Here's how the part is built. I have some questions about the finished solid (model axes, mm). Face numbers are marked on the shaded views. A direction names the side the tool comes from. Give positions to 0.01 mm unless a question says otherwise; leave off trailing zeros. Write each loop counter-clockwise with the first axis right and the second up, starting at its lowest first coordinate (ties: lowest second). Pieces come first, ordered by that corner, then holes. Notation, with made-up numbers: (67, 45.5) -> (122, 45.5) arc R19 cw to (122, 49.5) -> close; hole circle Ø4 at (-10, 45). An arc over 180 degrees is marked (long way). Return JSON: item names as keys, results as strings.
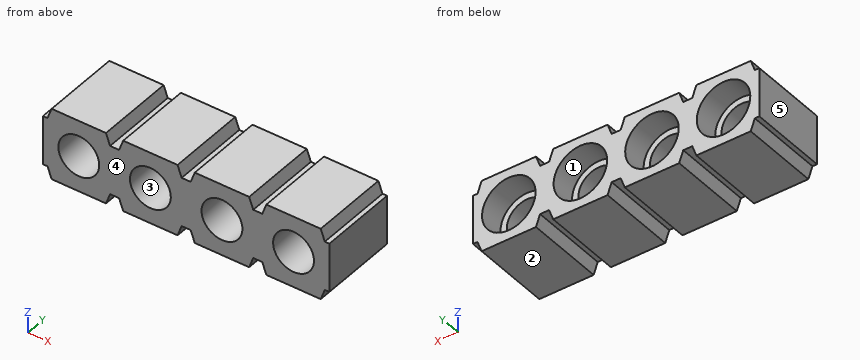
from build123d import *

# Parameters (mm, degrees)
EXTRUDE1_DEPTH    = 2.794
HOLE1_D           = 1.45034
HOLE1_CBORE_D     = 1.89992
HOLE1_CBORE_DEPTH = 0.89408
EXTRUDE2_DEPTH    = 2.794
LPATTERN1_COUNT   = 4
LPATTERN1_PITCH   = 2.54
LPATTERN2_COUNT   = 63
LPATTERN2_PITCH   = 2.54


with BuildPart() as part:
    # Sketch1 → Extrude1 (new body)
    with BuildSketch(Plane(origin=(0, 0, 0), x_dir=(1, 0, 0), z_dir=(0, 1, 0))):
        Polygon((9.854373708, 0.40005), (9.694353708, 0.40005), (9.548747416, 0), (0, 0), (-0.145606292, 0.40005), (-0.305626292, 0.40005), (-0.305626292, 2.13995), (-0.145606292, 2.13995), (0, 2.54), (9.548747416, 2.54), (9.694353708, 2.13995), (9.854373708, 2.13995), align=None)
    extrude(amount=-EXTRUDE1_DEPTH)

    # Hole1 (through all)
    with Locations(Plane(origin=(0.964373708, 0, -1.27), x_dir=(0, 0, 1), z_dir=(0, 1, 0))):
        with Locations((0, 0)):
            hole1 = CounterBoreHole(HOLE1_D / 2, HOLE1_CBORE_D / 2, HOLE1_CBORE_DEPTH)

    # Sketch4 → Extrude2 (cut)
    with BuildSketch(Plane(origin=(0, 0, 0), x_dir=(1, 0, 0), z_dir=(0, 1, 0))):
        Polygon((1.928772816, 0), (2.5399746, 0), (2.394368308, 0.40005), (2.074379108, 0.40005), align=None)
        Polygon((2.074379108, 2.13995), (2.394368308, 2.13995), (2.5399746, 2.54), (1.928772816, 2.54), align=None)
    extrude2 = extrude(amount=-EXTRUDE2_DEPTH, mode=Mode.SUBTRACT)

    # LPattern1: Hole1 ×4
    with Locations(*[(i * LPATTERN1_PITCH, 0, 0) for i in range(1, LPATTERN1_COUNT)]):
        add(hole1, mode=Mode.SUBTRACT)

    # LPattern2: Extrude2 ×63
    with Locations(*[(i * LPATTERN2_PITCH, 0, 0) for i in range(1, LPATTERN2_COUNT)]):
        add(extrude2, mode=Mode.SUBTRACT)


solid = part.part
1. For pin 1 Ø1.5 at (x, z) = (1, -1.5) entering from +Y; pin 2 Ø0.9 at (x, z) = (8.58, -1.27) entering from +Y, each with a flat end and sliding along its axis, tell me the tip position at first contact or that it passes through.
Taken from the geometry:
{"pin 1": "stops at y = 0", "pin 2": "passes through"}
2. If I drill on line 1 (X direction, y = -0.7, z = -1.27); line 2 (X direction, y = -2.05, z = -1.27); line 3 (X direction, y = -2.6, z = -2.3), over which ranges is the centre line in solid material (lowest first)? Write a range as [from, to].
Taken from the geometry:
{"line 1": "x = [-0.31, 0.01], [1.91, 2.55], [4.45, 5.09], [6.99, 7.63], [9.53, 9.85]", "line 2": "x = [-0.31, 0.24], [1.69, 2.78], [4.23, 5.32], [6.77, 7.86], [9.31, 9.85]", "line 3": "x = [-0.09, 2.02], [2.45, 4.56], [4.99, 7.1], [7.53, 9.64]"}
3. Which directions (+Z, -Z, +X, -X, +Y, -Y) give clear straight access to the entire face, cutting with the end or side of a thin tool? Please do the marked faces 1 and 2.
Taken from the geometry:
{"face 1": "+Y", "face 2": "-Z, +X, -X, +Y, -Y"}
4. Suppose I cut it at D-D, the plane x = 0.5. List the corners of the cut face in (y, z) for me, and give its area (3 significant figures).
Taken from the geometry:
{"outline": "(-2.79, -2.54) -> (0, -2.54) -> (0, -2.1) -> (-0.89, -2.1) -> (-0.89, -1.83) -> (-2.79, -1.83) -> close; (-2.79, -0.71) -> (-0.89, -0.71) -> (-0.89, -0.44) -> (0, -0.44) -> (0, 0) -> (-2.79, 0) -> close", "area": "3.50 mm²"}
5. Suppose I cut it at C-C, the plane z = -1.27. Count the separate pieces of the cut face and the enclosed holes in it, and give its area (3 significant figures).
Taken from the geometry:
{"separate pieces": "5", "enclosed holes": "0", "area": "10.6 mm²"}
6. Suppose I cut it at B-B, the plane z = -0.15. List the corners of the cut face in (x, y) for me.
Taken from the geometry:
{"outline": "(-0.05, -2.79) -> (1.98, -2.79) -> (1.98, 0) -> (-0.05, 0) -> close; (2.49, -2.79) -> (4.52, -2.79) -> (4.52, 0) -> (2.49, 0) -> close; (5.03, -2.79) -> (7.06, -2.79) -> (7.06, 0) -> (5.03, 0) -> close; (7.57, -2.79) -> (9.6, -2.79) -> (9.6, 0) -> (7.57, 0) -> close"}
7. If we mould it in two halves opening along X, with no side actions, what happens to the marked faces 3, 4 and 5? For each: released by +X, released by -X, zero draft, split by the parting line, or undercut.
Taken from the geometry:
{"face 3": "undercut", "face 4": "zero draft", "face 5": "released by -X"}
8. Suppose I cut it at A-A, the plane x = 8.75. List the corners of the cut face in (y, z) for me, and give its area (3 significant figures).
Taken from the geometry:
{"outline": "(-2.79, -2.54) -> (0, -2.54) -> (0, -2.21) -> (-0.89, -2.21) -> (-0.89, -1.98) -> (-2.79, -1.98) -> close; (-2.79, -0.56) -> (-0.89, -0.56) -> (-0.89, -0.33) -> (0, -0.33) -> (0, 0) -> (-2.79, 0) -> close", "area": "2.74 mm²"}
